```python
from build123d import *

# Parameters (mm, degrees)
SKETCH1_R           = 3.175
BOSS_EXTRUDE2_DEPTH = 3.175


with BuildPart() as part:
    # Sketch1 → Boss-Extrude2 (new body)
    with BuildSketch(Plane(origin=(0, 0, 0), x_dir=(1, 0, 0), z_dir=(0, 1, 0))):
        with BuildLine():
            ThreePointArc((88.862359447, -0.977063577), (85.519300066, 8.627899298), (76.2, 12.7))
            Line((76.2, 12.7), (0, 12.7))
            ThreePointArc((0, 12.7), (-10.244681695, 7.505764249), (-12.109317419, -3.828110715))
            Line((-12.109317419, -3.828110715), (49.140454024, -197.577189418))
            ThreePointArc((49.140454024, -197.577189418), (62.701866935, -206.365790583), (73.91213089, -194.726142279))
            Line((73.91213089, -194.726142279), (88.862359447, -0.977063577))
        make_face()
        Circle(SKETCH1_R, mode=Mode.SUBTRACT)
        Polygon((17.334338412, -12.7), (62.482279527, -12.7), (53.624378759, -127.494908088), align=None, mode=Mode.SUBTRACT)
        with Locations((61.249771443, -193.749078703)):
            Circle(SKETCH1_R, mode=Mode.SUBTRACT)
        with Locations((76.2, 0)):
            Circle(SKETCH1_R, mode=Mode.SUBTRACT)
    extrude(amount=BOSS_EXTRUDE2_DEPTH)


solid = part.part
```
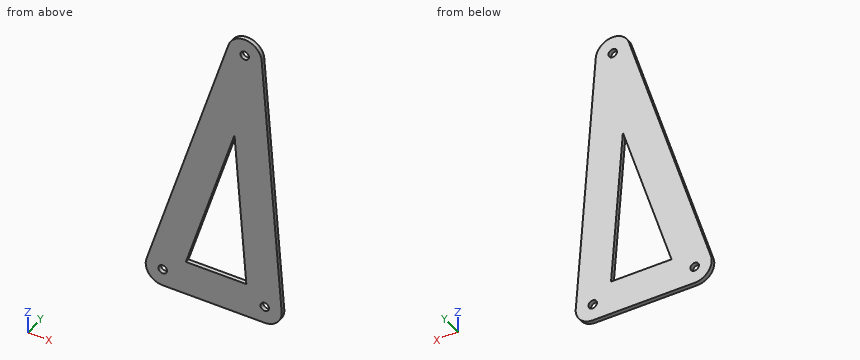
Here's how the part is built. I have some questions about the finished solid (model axes, mm). Coordinates: 2 decimals unless noted, no trailing zeros. Loops run counter-clockwise (first coordinate to the right, second up) from the corner with the lowest first, then second, coordinate; pieces in that order, holes last. Notation, with made-up numbers: M 59,-22 L 115,-22 A34 cw 115,15 Z; hole C 84.5,22.5 d3. An arc over 180 degrees is marked long. One line per item, written item: value.
1. Will these pins go through, and if not, where does the flat tip stop? pin 1 Ø6 at (x, z) = (30.5, 74.5) entering from -Y; pin 2 Ø1 at (y, z) = (1, 110) entering from +X.
Geometry says:
pin 1: stops at y = 0
pin 2: stops at x = 80.49
2. Please list where these lines run through material, in increasing order: probe 1 along X at (y, z) = (2.3, 0) (3 decimals); probe 2 along X at (y, z) = (2.5, 0.5); probe 3 along X at (y, z) = (1.3, 83.5).
Geometry says:
probe 1: x = -12.7 to -3.175, 3.175 to 73.025, 79.375 to 88.9
probe 2: x = -12.69 to -3.14, 3.14 to 73.06, 79.34 to 88.89
probe 3: x = 13.08 to 39.72, 57.02 to 82.49
3. Imagine slicing it at B-B (z = 122.5). List the corners of the cut face in (x, y) for me (3 decimals).
Geometry says:
outline: M 25.406,0 L 52.045,0 L 52.045,3.175 L 25.406,3.175 Z; M 54.01,0 L 79.485,0 L 79.485,3.175 L 54.01,3.175 Z
4. Imagine slicing it at D-D (x = 70.5). List the corners of the cut face in (y, z) for me (3 decimals), and give its area (3 significant figures).
Geometry says:
outline: M 0,-12.7 L 3.175,-12.7 L 3.175,202.451 L 0,202.451 Z
area: 683 mm2
5. Imagine slicing it at A-A (y = 1.05). List the corners of the cut face in (x, z) for me (3 decimals), and give its area (3 significant figures).
Geometry says:
outline: M -12.109,3.828 A12.7 ccw 0,-12.7 L 76.2,-12.7 A12.7 ccw 88.862,0.977 L 73.912,194.726 A12.7 ccw 49.14,197.577 Z; hole C 0,0 d6.35; hole M 17.334,12.7 L 62.482,12.7 L 53.624,127.495 Z; hole C 61.25,193.749 d6.35; hole C 76.2,0 d6.35
area: 11,200 mm2
6. Imagine slicing it at C-C (x = 33). List the corners of the cut face in (y, z) for me (3 decimals).
Geometry says:
outline: M 0,-12.7 L 3.175,-12.7 L 3.175,12.7 L 0,12.7 Z; M 0,62.255 L 3.175,62.255 L 3.175,146.521 L 0,146.521 Z
